from build123d import *

# Parameters (mm, degrees)
SKETCH2_W            = 111.76
SKETCH2_H            = 40.64
SKETCH2_R            = 3.175
BOSS_EXTRUDE13_DEPTH = 4.953
BOSS_EXTRUDE14_DEPTH = 4.953


with BuildPart() as part:
    # Sketch2 → Boss-Extrude13 (new body)
    with BuildSketch(Plane.XY):
        Rectangle(SKETCH2_W, SKETCH2_H)
        with Locations((50.8, 0)):
            Circle(SKETCH2_R, mode=Mode.SUBTRACT)
        with Locations((-50.8, 0)):
            Circle(SKETCH2_R, mode=Mode.SUBTRACT)
    extrude(amount=BOSS_EXTRUDE13_DEPTH)

    # Sketch3 → Boss-Extrude14 (add)
    with BuildSketch(Plane.XY.offset(4.953)):
        with BuildLine():
            Line((27.305, -19.05), (-27.305, -19.05))
            ThreePointArc((-27.305, -19.05), (-46.355, 0), (-27.305, 19.05))
            Line((-27.305, 19.05), (27.305, 19.05))
            ThreePointArc((27.305, 19.05), (46.355, 0), (27.305, -19.05))
        make_face()
    extrude(amount=BOSS_EXTRUDE14_DEPTH)


solid = part.part
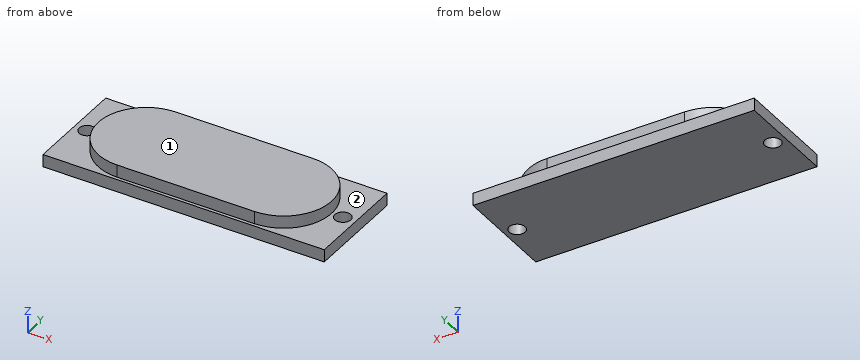
Model file for the job. Use its own axes, mm. Face numbers are marked on the shaded views. A direction names the side the tool comes from. Give positions to 0.01 mm unless a question says otherwise; leave off trailing zeros. Write each loop counter-clockwise with the first axis right and the second up, starting at its lowest first coordinate (ties: lowest second). Pieces come first, ordered by that corner, then holes. Notation, with made-up numbers: (-24.5, -35.5) - (33.5, -35.5) arc R20 ccw to (33.5, -4.5) - close; hole circle Ø6 at (33.25, 32.25). An arc over 180 degrees is marked (long way). Answer as CSV lines item,"result".
1. Band-saw the part on B-B (x = -50.8). Write the cut outline in (y, z) (3 decimals), and give its area (3 significant figures).
Responses:
outline,"(-20.32, 0) - (-3.175, 0) - (-3.175, 4.953) - (-20.32, 4.953) - close; (3.175, 0) - (20.32, 0) - (20.32, 4.953) - (3.175, 4.953) - close"
area,"170 mm2"
2. 3-axis set-ups, long thin cutter, end or side, ignore diameter. For the marked faces 1 and 2: which of +Z, -Z, +X, -X, +Y, -Y reach the whole face in a straight line?
Responses:
face 1,"+Z, +X, -X, +Y, -Y"
face 2,"+Z"
3. Band-saw the part on C-C (x = -13.5). Write the cut outline in (y, z).
Responses:
outline,"(-20.32, 0) - (20.32, 0) - (20.32, 4.95) - (19.05, 4.95) - (19.05, 9.91) - (-19.05, 9.91) - (-19.05, 4.95) - (-20.32, 4.95) - close"
4. Band-saw the part on D-D (y = 5.5). Write the cut outline in (x, z), and give its area (3 significant figures).
Responses:
outline,"(-55.88, 0) - (55.88, 0) - (55.88, 4.95) - (45.54, 4.95) - (45.54, 9.91) - (-45.54, 9.91) - (-45.54, 4.95) - (-55.88, 4.95) - close"
area,"1,000 mm2"
5. Band-saw the part on A-A (y = 0). Write the cut outline in (x, z) (3 decimals).
Responses:
outline,"(-55.88, 0) - (-53.975, 0) - (-53.975, 4.953) - (-55.88, 4.953) - close; (-47.625, 0) - (47.625, 0) - (47.625, 4.953) - (46.355, 4.953) - (46.355, 9.906) - (-46.355, 9.906) - (-46.355, 4.953) - (-47.625, 4.953) - close; (53.975, 0) - (55.88, 0) - (55.88, 4.953) - (53.975, 4.953) - close"
6. Drill centre lines: L1, parallel to Y at x = 50.8, z = 1 (3 decimals); L2, parallel to X at y = 0.5, z = 3.75; L3, parallel to X at y = -1, z = 2.5. Where is each one in solid material? Low to high. Write a range as [from, to].
Responses:
L1,"y = [-20.32, -3.175], [3.175, 20.32]"
L2,"x = [-55.88, -53.94], [-47.66, 47.66], [53.94, 55.88]"
L3,"x = [-55.88, -53.81], [-47.79, 47.79], [53.81, 55.88]"
7. Pin check, flat tips, straight feed: pin 1 (8.5 mm diameter, centred on x = 50.8, y = 0, fed in from -Z); pin 2 (4 mm diameter, centred on x = -50.8, y = 0, fed in from +Z); pin 3 (1.5 mm diameter, centred on x = -12.5, z = 8.5, fed in from -Y); pin 4 (5 mm diameter, centred on x = -27.5, z = 7.5, fed in from +Y). Stop position of each tip, or through.
Responses:
pin 1,"stops at z = 0"
pin 2,"passes through"
pin 3,"stops at y = -19.05"
pin 4,"stops at y = 19.05"
